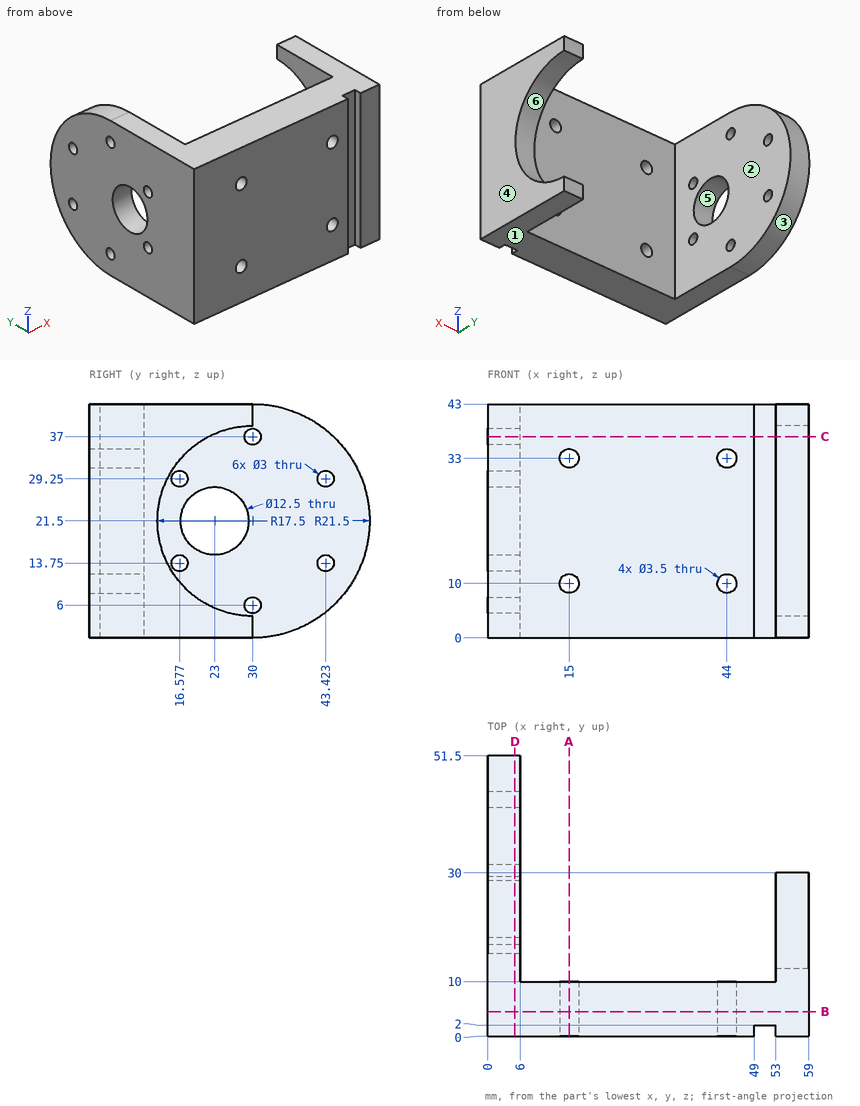
Here's the drawing with two shaded views (mm, measured from the low corner). I have some questions. A direction names the side the tool comes from. Round coordinates to 2 decimals unless told otherwise and drop trailing zeros. Loops run counter-clockwise (first coordinate to the right, second up) from the corner with the lowest first, then second, coordinate; pieces in that order, holes last. Notation, with made-up numbers: (88, -6) -> (136, -6) arc R27 cw to (136, 29) -> close; hole circle Ø5 at (-38.75, -22.5). An arc over 180 degrees is marked (long way). Answer as CSV lines item,"result". Start each with the question number.
1. I need wall thicknesses on probe 1 along X at (y, z) = (29.5, 2); probe 2 along Y at (x, z) = (1.75, 29.25) (1 decimal); probe 3 along Y at (x, z) = (21, 3.5). Which ranges of each line are inside material? Lowest first, please. Write a range as from..to.
2. Imagine slicing it at D-D on x = 5. Write out the boundary of the cut face in (y, z), plus the area to 3 significant figures.
3. Imagine slicing it at A-A on x = 15. Write out the boundary of the cut face in (y, z), plus the area to 3 significant figures.
4. For the marked faces 1 and 2, which set-ups out of +Z, -Z, +X, -X, +Y, -Y let a thin tool reach every point of the face, with its end or its side?
5. Imagine slicing it at C-C on z = 37. Write out the boundary of the cut face in (x, y).
6. Imagine slicing it at B-B on y = 4.5. Write out the boundary of the cut face in (x, z), plus the area to 3 significant figures.
7. I'm going to push flat-ended pins straight in: P1, Ø20, axis at y = 23, z = 21.5, coming from the +X side; P2, Ø2, axis at x = 42.5, z = 15, coming from the -Y side; P3, Ø6, axis at x = 38, z = 7.5, coming from the +Y side. Where does each tip first touch, or does it pass through?
8. If we mould it in two halves opening along Z, with no side actions, what happens to the marked faces 3, 4, 5 and 6? For each: pulls with the +Z half, pulls with the -Z half, needs draft (parallel to the pull), parting line crosses it, or undercut.
Solution:
1,probe 1,"0..6, 53..59"
1,probe 2,"0..15.1, 18.1..41.9, 44.9..50.1"
1,probe 3,"0..10"
2,outline,"(0, 0) -> (30, 0) arc R21.5 ccw to (30, 43) -> (0, 43) -> close; hole circle Ø3 at (16.58, 13.75); hole circle Ø3 at (16.58, 29.25); hole circle Ø12.5 at (23, 21.5); hole circle Ø3 at (30, 6); hole circle Ø3 at (30, 37); hole circle Ø3 at (43.42, 13.75); hole circle Ø3 at (43.42, 29.25)"
2,area,"1,850 mm²"
3,outline,"(0, 0) -> (10, 0) -> (10, 8.25) -> (0, 8.25) -> close; (0, 11.75) -> (10, 11.75) -> (10, 31.25) -> (0, 31.25) -> close; (0, 34.75) -> (10, 34.75) -> (10, 43) -> (0, 43) -> close"
3,area,"360 mm²"
4,face 1,"-Z, +X, -X, +Y, -Y"
4,face 2,"+Z, -Z, +Y"
5,outline,"(0, 0) -> (49, 0) -> (49, 2) -> (53, 2) -> (53, 0) -> (59, 0) -> (59, 21.88) -> (53, 21.88) -> (53, 10) -> (6, 10) -> (6, 28.5) -> (0, 28.5) -> close; (0, 31.5) -> (6, 31.5) -> (6, 44.9) -> (0, 44.9) -> close"
6,outline,"(0, 0) -> (59, 0) -> (59, 43) -> (0, 43) -> close; hole circle Ø3.5 at (15, 10); hole circle Ø3.5 at (15, 33); hole circle Ø3.5 at (44, 10); hole circle Ø3.5 at (44, 33)"
6,area,"2,500 mm²"
7,P1,"x = 6"
7,P2,"y = 0"
7,P3,"y = 10"
8,face 3,"parting line crosses it"
8,face 4,"needs draft"
8,face 5,"undercut"
8,face 6,"undercut"
